Source: CAD feature listing. Evaluate the final solid. Frame: model axes, mm. Face numbers are marked on the shaded views. A direction names the side the tool comes from. Coordinates: 2 decimals unless noted, no trailing zeros. Write each loop counter-clockwise with the first axis right and the second up, starting at its lowest first coordinate (ties: lowest second). Pieces come first, ordered by that corner, then holes. Notation, with made-up numbers: M 65,40 L 102,40 A30 ccw 102,74 Z; hole C -37.75,5.5 d7. An arc over 180 degrees is marked long. Answer as CSV lines item,"result". Start each with the question number.
1. Contact query for flat-ended pins moving along their axis: pin 1 Ø11 at (x, y) = (-2.5, 27.5) entering from -Z; pin 2 Ø5 at (y, z) = (14, -1) entering from +X; pin 3 Ø5 at (x, y) = (1, 25) entering from +Z. Output: stop coordinate, or through.
2. Section B-B on x = -26. Return the cut outline in (y, z).
3. Mould query, pull axis Y, two halves, no side actions, for the marked faces 1, 2 and 3. Classes: pulls with the +Y half, pulls with the -Y half, needs draft (parallel to the pull), parting line crosses it, or undercut.
4. Section A-A on z = 0. Count the separate pieces of the cut face and the enclosed holes in it, plus the area to 3 significant figures.
5. Reachability of the marked faces 4, 5 and 6 from +Z, -Z, +X, -X, +Y, -Y: full face, straight path, thin tool, end or side. Return the list, or none.
6. Section D-D on y = 23. Return the cut outline in (x, z).
7. Line query: probe 1 along X at (y, z) = (40.5, 0); probe 2 along X at (y, z) = (1.8, 0); probe 3 along Y at (x, z) = (1, 4). Output: solid intervals per line, ascending. Write a range as [from, to].
8. Section C-C on x = 3.5. Return the cut outline in (y, z), plus the area to 3 significant figures.
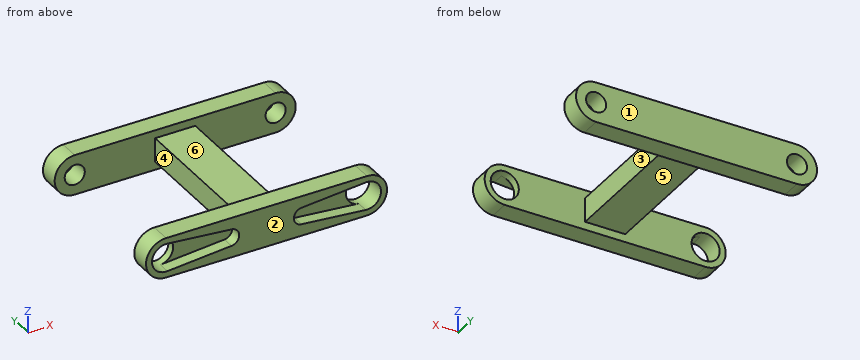
```python
from build123d import *

# Parameters (mm, degrees)
SKETCH2_W           = 60
SKETCH2_H           = 10
BOSS_EXTRUDE1_DEPTH = 5
FILLET1_RADIUS      = 5
FILLET1_LENGTH      = 5
FILLET2_RADIUS      = 5
FILLET2_LENGTH      = 5
SKETCH11_W          = 4.99996664
SKETCH11_H          = 10
BOSS_EXTRUDE3_DEPTH = 34
SKETCH12_W          = 2
SKETCH12_H          = 34
CUT_EXTRUDE6_DEPTH  = 18
BOSS_EXTRUDE4_DEPTH = 5
SKETCH14_R          = 2.5
CUT_EXTRUDE7_DEPTH  = 5
SKETCH15_R          = 3.5
CUT_EXTRUDE8_DEPTH  = 5
CUT_EXTRUDE10_DEPTH = 3


with BuildPart() as part:
    # Sketch2 → Boss-Extrude1 (new body)
    with BuildSketch(Plane(origin=(0, 0, 0), x_dir=(1, 0, 0), z_dir=(0, 1, 0))):
        Rectangle(SKETCH2_W, SKETCH2_H)
    extrude(amount=BOSS_EXTRUDE1_DEPTH)

    # Fillet1: full round fillet: the end face becomes a half cylinder, R = half its width
    fillet1_face = Plane((-30, 2.5, 0), x_dir=(0, 1, 0), z_dir=(-1, 0, 0))  # on the end face: x along it, z out of the body
    fillet1_slab = fillet1_face.offset(-FILLET1_RADIUS / 2) * Box(FILLET1_LENGTH, 2 * FILLET1_RADIUS, FILLET1_RADIUS, mode=Mode.PRIVATE)  # the body's end, R deep
    fillet1_round = Plane((-25, 2.5, 0), x_dir=(-1, 0, 0), z_dir=(0, 1, 0)) * Cylinder(FILLET1_RADIUS, FILLET1_LENGTH, mode=Mode.PRIVATE)  # its axis R under the face
    add(fillet1_slab - fillet1_round, mode=Mode.SUBTRACT)

    # Fillet2: full round fillet: the end face becomes a half cylinder, R = half its width
    fillet2_face = Plane((30, 2.5, 0), x_dir=(0, -1, 0), z_dir=(1, 0, 0))  # on the end face: x along it, z out of the body
    fillet2_slab = fillet2_face.offset(-FILLET2_RADIUS / 2) * Box(FILLET2_LENGTH, 2 * FILLET2_RADIUS, FILLET2_RADIUS, mode=Mode.PRIVATE)  # the body's end, R deep
    fillet2_round = Plane((25, 2.5, 0), x_dir=(1, 0, 0), z_dir=(0, -1, 0)) * Cylinder(FILLET2_RADIUS, FILLET2_LENGTH, mode=Mode.PRIVATE)  # its axis R under the face
    add(fillet2_slab - fillet2_round, mode=Mode.SUBTRACT)

    # Sketch11 → Boss-Extrude3 (add)
    with BuildSketch(Plane(origin=(0, 5, 0), x_dir=(1, 0, 0), z_dir=(0, 1, 0))):
        with Locations((2.49998332, 0)):
            Rectangle(SKETCH11_W, SKETCH11_H)
        Polygon((0, -5), (0, 5), (-4.99996664, 4.981735201), (-4.99996664, -5), align=None)
    extrude(amount=BOSS_EXTRUDE3_DEPTH)

    # Sketch12 → Cut-Extrude6 (cut)
    with BuildSketch(Plane(origin=(4.99996664, 0, 0), x_dir=(0, 0, -1), z_dir=(1, 0, 0))):
        with Locations((-4, 22)):
            Rectangle(SKETCH12_W, SKETCH12_H)
        with Locations((4, 22)):
            Rectangle(SKETCH12_W, SKETCH12_H)
    extrude(amount=-CUT_EXTRUDE6_DEPTH, mode=Mode.SUBTRACT)

    # Sketch13 → Boss-Extrude4 (add)
    with BuildSketch(Plane(origin=(0, 39, 0), x_dir=(1, 0, 0), z_dir=(0, 1, 0))):
        with BuildLine():
            Line((25, 5), (-25, 5))
            ThreePointArc((-25, 5), (-30, 0), (-25, -5))
            Line((-25, -5), (25, -5))
            ThreePointArc((25, -5), (30, 0), (25, 5))
        make_face()
    extrude(amount=BOSS_EXTRUDE4_DEPTH)

    # Sketch14 → Cut-Extrude7 (cut)
    with BuildSketch(Plane(origin=(0, 44, 0), x_dir=(1, 0, 0), z_dir=(0, 1, 0))):
        with Locations(Location((-25, 0, 0), (0, 0, 270))):
            Circle(SKETCH14_R)
        with Locations(Location((25, 0, 0), (0, 0, 90))):
            Circle(SKETCH14_R)
    extrude(amount=-CUT_EXTRUDE7_DEPTH, mode=Mode.SUBTRACT)

    # Sketch15 → Cut-Extrude8 (cut)
    with BuildSketch(Plane.XZ):
        with Locations(Location((-25, 0, 0), (0, 0, 270))):
            Circle(SKETCH15_R)
        with Locations(Location((25, 0, 0), (0, 0, 270))):
            Circle(SKETCH15_R)
    extrude(amount=-CUT_EXTRUDE8_DEPTH, mode=Mode.SUBTRACT)

    # Sketch18 → Cut-Extrude10 (cut)
    with BuildSketch(Plane.XZ):
        with BuildLine():
            ThreePointArc((-24.695652174, 3.486742377), (-21.5, 0), (-24.695652174, -3.486742377))
            Line((-24.695652174, -3.486742377), (-8.717391304, -2.092045426))
            ThreePointArc((-8.717391304, -2.092045426), (-6.8, 0), (-8.717391304, 2.092045426))
            Line((-8.717391304, 2.092045426), (-24.695652174, 3.486742377))
        make_face()
        with BuildLine():
            Line((8.717391304, -2.092045426), (24.695652174, -3.486742377))
            ThreePointArc((24.695652174, -3.486742377), (21.5, 0), (24.695652174, 3.486742377))
            Line((24.695652174, 3.486742377), (8.717391304, 2.092045426))
            ThreePointArc((8.717391304, 2.092045426), (6.8, 0), (8.717391304, -2.092045426))
        make_face()
    extrude(amount=-CUT_EXTRUDE10_DEPTH, mode=Mode.SUBTRACT)


solid = part.part
```
Values:
1,pin 1,"z = -3"
1,pin 2,"x = 5"
1,pin 3,"z = 3"
2,outline,"M 0,-4.9 L 5,-4.9 L 5,-3.35 L 0,-3.35 Z; M 0,3.35 L 5,3.35 L 5,4.9 L 0,4.9 Z; M 39,-4.9 L 44,-4.9 L 44,-2.29 L 39,-2.29 Z; M 39,2.29 L 44,2.29 L 44,4.9 L 39,4.9 Z"
3,face 1,"pulls with the +Y half"
3,face 2,"pulls with the -Y half"
3,face 3,"undercut"
4,separate pieces,"5"
4,enclosed holes,"0"
4,area,"732 mm²"
5,face 4,"+Z, -Z, -X"
5,face 5,"-Z, +X, -X"
5,face 6,"+Z, +X, -X"
6,outline,"M -5,-3 L 5,-3 L 5,3 L -5,3 Z"
7,probe 1,"[-30, -27.5], [-22.5, 22.5], [27.5, 30]"
7,probe 2,"[-30, -28.5], [-6.8, 6.8], [28.5, 30]"
7,probe 3,"[0, 5], [39, 44]"
8,outline,"M 0,-5 L 5,-5 L 5,-3 L 39,-3 L 39,-5 L 44,-5 L 44,5 L 39,5 L 39,3 L 5,3 L 5,5 L 0,5 Z"
8,area,"304 mm²"
